```python
from build123d import *

# Parameters (mm, degrees)
F0_W      = 57
F0_H      = 57
F1_DEPTH  = 10
F2_W      = 5
F2_H      = 47
F2_W_2    = 47
F2_H_2    = 5
F3_DEPTH  = 85.0000008941
F4_W      = 30
F4_H      = 13
F5_DEPTH  = 30
F6_SIZE   = 5
F7_R      = 7.5
F8_DEPTH  = 5
F9_R      = 5
F10_DEPTH = 50


with BuildPart() as f1:
    # F0 (on Front) → F1 (new body)
    with BuildSketch(Plane.XZ):
        Rectangle(F0_W, F0_H)
    extrude(amount=F1_DEPTH)

    # F2 (on face) → F3 (join)
    with BuildSketch(Plane(origin=(0, 0, 0), x_dir=(-1, 0, 0), z_dir=(0, 1, 0))):
        with Locations((-26, 0)):
            Rectangle(F2_W, F2_H)
        with Locations((0, 26)):
            Rectangle(F2_W_2, F2_H_2)
        with Locations((26, 0)):
            Rectangle(F2_W, F2_H)
        Rectangle(F2_W_2, F2_H)
        with Locations((0, -26)):
            Rectangle(F2_W_2, F2_H_2)
    extrude(amount=-F3_DEPTH)

    # F4 (on face) → F5 (join)
    with BuildSketch(Plane.XZ.offset(85.0000008941)):
        with Locations((0, 35)):
            Rectangle(F4_W, F4_H)
    extrude(amount=-F5_DEPTH)

    # F6
    f6_edges = [f1.edges().sort_by_distance(p)[0] for p in [
        (15, -70.000001, 41.5),
        (-15, -70.000001, 41.5),
    ]]
    chamfer(f6_edges, length=F6_SIZE)

    # F7 (on face) → F8 (cut)
    with BuildSketch(Plane(origin=(0, 0, 0), x_dir=(-1, 0, 0), z_dir=(0, 1, 0))):
        Circle(F7_R)
    extrude(amount=-F8_DEPTH, mode=Mode.SUBTRACT)

    # F9 (on face) → F10 (join)
    with BuildSketch(Plane(origin=(0, -5, 0), x_dir=(-1, 0, 0), z_dir=(0, 1, 0))):
        Circle(F9_R)
    extrude(amount=F10_DEPTH)


solid = f1.part
```
Part model, mm, in its own coordinate system. A direction names the side the tool comes from. Give positions to 0.01 mm unless a question says otherwise; leave off trailing zeros. Order: outer loops, then holes, each group sorted by start corner. A loop starts at its lowest first (then second) coordinate and runs counter-clockwise, first axis right, second up. Notation, with made-up numbers: M 28,61.5 L 47,61.5 A29 ccw 47,86.5 Z; hole C -22.75,-29 d4. An arc over 180 degrees is marked long. Use a Markdown table: item, result. Add a question column.
(1) Saw through at A-A, the plane z = 0. Give the cut face in (x, y).
(2) Drop flat-ended pins along their axis: P1, Ø5.5, axis at x = 27, y = -44.5, coming from the +Z side; P2, Ø5.5, axis at y = -46, z = 26.5, coming from the +X side; P3, Ø1.5, axis at x = 25, z = -26, coming from the -Y side; P4, Ø8, axis at x = -4, z = -4.5, coming from the +Y side. Give the stop position or say it passes through.
(3) Saw through at D-D, the plane y = -45. Give the cut face in (x, z), and give its area (3 significant figures).
(4) Saw through at C-C, the plane y = -59. Give the cut face in (x, z).
(5) Probe line 1 along Z through (x, y) = (0, -3.85); line 2 along X through (y, z) = (-3, -4); line 3 along Y through (x, z) = (21, -17). List the from-to ranges inside material, lowest first. Write a range as [from, to].
(6) Saw through at B-B, the plane x = 0. Give the cut face in (y, z), and give its area (3 significant figures).
(7) 3-axis set-ups, long thin cutter, end or side, ignore diameter. For faces 1 (the face through (0, -55, 35)), 2 (the face through (-26, -47, -23.5)), 3 (the face through (23.5, -47, 26)): which of +Z, -Z, +X, -X, +Y, -Y reach the whole face in a straight line?
Answer key:
| question | item | result |
|---|---|---|
| 1 | outline | M -28.5,-85 L 28.5,-85 L 28.5,0 L 7.5,0 L 7.5,-5 L 5,-5 L 5,45 L -5,45 L -5,-5 L -7.5,-5 L -7.5,0 L -28.5,0 Z |
| 2 | P1 | z = 23.5 |
| 2 | P2 | x = 23.5 |
| 2 | P3 | y = -10 |
| 2 | P4 | y = 45 |
| 3 | outline | M -28.5,-23.5 L -23.5,-23.5 L -23.5,-28.5 L 23.5,-28.5 L 23.5,-23.5 L 28.5,-23.5 L 28.5,23.5 L 23.5,23.5 L 23.5,28.5 L -23.5,28.5 L -23.5,23.5 L -28.5,23.5 Z |
| 3 | area | 3,150 mm^2 |
| 4 | outline | M -28.5,-23.5 L -23.5,-23.5 L -23.5,-28.5 L 23.5,-28.5 L 23.5,-23.5 L 28.5,-23.5 L 28.5,23.5 L 23.5,23.5 L 23.5,28.5 L 15,28.5 L 15,36.5 L 10,41.5 L -10,41.5 L -15,36.5 L -15,28.5 L -23.5,28.5 L -23.5,23.5 L -28.5,23.5 Z |
| 5 | line 1 | [-28.5, -7.5], [-5, 5], [7.5, 28.5] |
| 5 | line 2 | [-28.5, -6.34], [-3, 3], [6.34, 28.5] |
| 5 | line 3 | [-85, 0] |
| 6 | outline | M -85,-28.5 L 0,-28.5 L 0,-7.5 L -5,-7.5 L -5,-5 L 45,-5 L 45,5 L -5,5 L -5,7.5 L 0,7.5 L 0,28.5 L -55,28.5 L -55,41.5 L -85,41.5 Z |
| 6 | area | 5,660 mm^2 |
| 7 | face 1 | +Z, +X, -X, +Y |
| 7 | face 2 | -Z, -X, -Y |
| 7 | face 3 | +Z, +X, -Y |
